Source: CAD feature listing. Evaluate the final solid. Frame: model axes, mm. Face numbers are marked on the shaded views. Give positions to 0.01 mm unless a question says otherwise; leave off trailing zeros. Order: outer loops, then holes, each group sorted by start corner. A loop starts at its lowest first (then second) coordinate and runs counter-clockwise, first axis right, second up. Notation, with made-up numbers: M 40,69 L 76,69 A17 ccw 76,85 Z; hole C 35.25,78 d9. An arc over 180 degrees is marked long. Return JSON: item names as keys, results as strings.
from build123d import *

# Parameters (mm, degrees)
SKETCH3_R               = 7
SKETCH3_R_2             = 4.15
BOSS_EXTRUDE1_DEPTH     = 16
SKETCH4_R               = 5
SKETCH4_R_2             = 3.2
BOSS_EXTRUDE2_DEPTH     = 8
CUT_EXTRUDE1_DEPTH      = 24.345235227
CUT_EXTRUDE1_DEPTH_BACK = 24.345235227


with BuildPart() as part:
    # Sketch3 → Boss-Extrude1 (new body)
    with BuildSketch(Plane(origin=(0, 0, 0), x_dir=(1, 0, 0), z_dir=(0, 1, 0))):
        with Locations(Location((0, 0, 0), (0, 0, 270))):
            Circle(SKETCH3_R)
        with Locations(Location((0, 0, 0), (0, 0, 270))):
            Circle(SKETCH3_R_2, mode=Mode.SUBTRACT)
    extrude(amount=BOSS_EXTRUDE1_DEPTH)

    # Sketch4 → Boss-Extrude2 (add, symmetric)
    with BuildSketch(Plane.XY):
        with Locations((-10, 5)):
            Circle(SKETCH4_R)
        with Locations((-10, 5)):
            Circle(SKETCH4_R_2, mode=Mode.SUBTRACT)
    extrude(amount=BOSS_EXTRUDE2_DEPTH, both=True)

    # Sketch4_2 → Cut-Extrude1 (cut, two sides: drawn at the far end of the back side and taken through both)
    with BuildSketch(Plane.XY.offset(-CUT_EXTRUDE1_DEPTH_BACK)):
        with BuildLine():
            ThreePointArc((-6.8, 5), (-6.85039685, 5.565685425), (-7, 6.113552873))
            Line((-7, 6.113552873), (-7, 3.886447127))
            ThreePointArc((-7, 3.886447127), (-6.85039685, 4.434314575), (-6.8, 5))
        make_face()
        with BuildLine():
            Line((-7, 3.886447127), (-7, 6.113552873))
            ThreePointArc((-7, 6.113552873), (-13.2, 5), (-7, 3.886447127))
        make_face()
    extrude(amount=CUT_EXTRUDE1_DEPTH + CUT_EXTRUDE1_DEPTH_BACK, mode=Mode.SUBTRACT)


solid = part.part
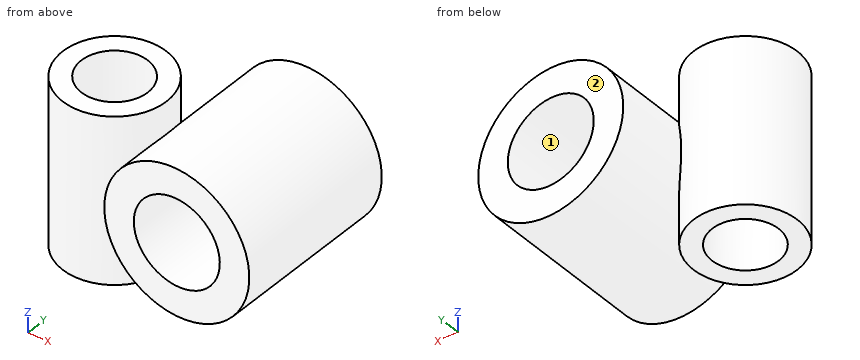
1. First-contact query: pin 1 (6 mm diameter, centred on y = 8.5, z = -1.5, fed in from -X); pin 2 (1.5 mm diameter, centred on x = -5.5, y = 12, fed in from +Z); pin 3 (6 mm diameter, centred on x = -5, y = 14, fed in from -Z). Flat tips, straight axial feed; report the tip coordinate or a pass-through.
Evaluation:
{"pin 1": "stops at x = -14.97", "pin 2": "stops at z = 5.14", "pin 3": "stops at z = -6.71"}
2. Section query A-A (z = 0). Return loops of the section in (x, y), then the cut area to 3 significant figures.
Evaluation:
{"outline": "M -7,0 L -4.15,0 L -4.15,16 L -7,16 L -7,9 A5 ccw long -7,1 Z; M 4.15,0 L 7,0 L 7,16 L 4.15,16 Z; hole C -10,5 d6.4", "area": "126 mm^2"}
3. Section query B-B (x = 0). Return loops of the section in (y, z).
Evaluation:
{"outline": "M 0,-7 L 16,-7 L 16,-4.15 L 0,-4.15 Z; M 0,4.15 L 16,4.15 L 16,7 L 0,7 Z"}
4. Draft query along X for the marked faces 1 and 2. Return one class per face: pulls with the +X half, pulls with the -X half, needs draft (parallel to the pull), parting line crosses it, or undercut.
Evaluation:
{"face 1": "undercut", "face 2": "needs draft"}
5. Section query C-C (z = 3.75). Return loops of the section in (x, y), then the cut area to 3 significant figures.
Evaluation:
{"outline": "M -5.91,0 L -1.78,0 L -1.78,16 L -5.91,16 L -5.91,7.88 A5 ccw long -5.91,2.12 Z; M 1.78,0 L 5.91,0 L 5.91,16 L 1.78,16 Z; hole C -10,5 d6.4", "area": "175 mm^2"}
6. Section query D-D (x = -10). Return loops of the section in (y, z), then the cut area to 3 significant figures.
Evaluation:
{"outline": "M 0,-8 L 1.8,-8 L 1.8,8 L 0,8 Z; M 8.2,-8 L 10,-8 L 10,8 L 8.2,8 Z", "area": "57.6 mm^2"}
7. Ray query, probe 1 along X at (y, z) = (4, 0); probe 2 along Y at (x, z) = (-10, -4.25); probe 3 along X at (y, z) = (6.75, -0.5). Return the intervals inside material, ascending.
Evaluation:
{"probe 1": "x = -14.9 to -13.04, -6.96 to -4.15, 4.15 to 7", "probe 2": "y = 0 to 1.8, 8.2 to 10", "probe 3": "x = -14.68 to -12.68, -7.32 to -4.12, 4.12 to 6.98"}
